```python
from build123d import *

# Parameters (mm, degrees)
SKETCH_1_W          = 80
SKETCH_1_H          = 50
EXTRUDE_1_DEPTH     = 2
SKETCH_5_W          = 2
SKETCH_5_H          = 50
EXTRUDE_2_DEPTH     = 2
SKETCH_2_W          = 30
SKETCH_2_H          = 4
SKETCH_2_W_2        = 35
SKETCH_2_H_2        = 16
CUT_EXTRUDE_1_DEPTH = 49.918299235
SKETCH_3_R          = 1.65
CUT_EXTRUDE_2_DEPTH = 49.918299235
SKETCH_6_W          = 1.5
SKETCH_6_H          = 4
CUT_EXTRUDE_4_DEPTH = 49.918299235
SKETCH_7_W          = 1.5
SKETCH_7_H          = 4
EXTRUDE_3_DEPTH     = 2
SKETCH_8_R          = 1.65
CUT_EXTRUDE_5_DEPTH = 49.918299235


with BuildPart() as part:
    # 草图1 → 凸台-拉伸1 (new body)
    with BuildSketch(Plane.XY):
        Rectangle(SKETCH_1_W, SKETCH_1_H)
    extrude(amount=EXTRUDE_1_DEPTH)

    # 草图5 → 凸台-拉伸2 (add)
    with BuildSketch(Plane.XY.offset(2)):
        with Locations((-41, 0)):
            Rectangle(SKETCH_5_W, SKETCH_5_H)
    extrude(amount=-EXTRUDE_2_DEPTH)

    # 草图2 → 切除-拉伸1 (cut, through all)
    with BuildSketch(Plane.XY.offset(2)):
        with Locations((0, -23)):
            Rectangle(SKETCH_2_W, SKETCH_2_H)
        with Locations((-0.5, -9)):
            Rectangle(SKETCH_2_W_2, SKETCH_2_H_2)
    extrude(amount=-CUT_EXTRUDE_1_DEPTH, mode=Mode.SUBTRACT)

    # 草图3 → 切除-拉伸2 (cut, through all)
    with BuildSketch(Plane.XY.offset(2)):
        with Locations((-39, -22)):
            Circle(SKETCH_3_R)
        with Locations((-19, -22)):
            Circle(SKETCH_3_R)
        with Locations(Location((17, -22, 0), (0, 0, 180))):
            Circle(SKETCH_3_R)
        with Locations(Location((37, -22, 0), (0, 0, 180))):
            Circle(SKETCH_3_R)
    extrude(amount=-CUT_EXTRUDE_2_DEPTH, mode=Mode.SUBTRACT)

    # 草图6 → 切除-拉伸4 (cut, through all)
    with BuildSketch(Plane.XY.offset(2)):
        with Locations((-15.75, -23)):
            Rectangle(SKETCH_6_W, SKETCH_6_H)
    extrude(amount=-CUT_EXTRUDE_4_DEPTH, mode=Mode.SUBTRACT)

    # 草图7 → 凸台-拉伸3 (add)
    with BuildSketch(Plane.XY.offset(2)):
        with Locations((14.25, -23)):
            Rectangle(SKETCH_7_W, SKETCH_7_H)
    extrude(amount=-EXTRUDE_3_DEPTH)

    # 草图8 → 切除-拉伸5 (cut, through all)
    with BuildSketch(Plane.XY.offset(2)):
        with Locations((-25, 11.5)):
            Circle(SKETCH_8_R)
        with Locations((-25, -8.5)):
            Circle(SKETCH_8_R)
        with Locations((25, -8.5)):
            Circle(SKETCH_8_R)
        with Locations((25, 11.5)):
            Circle(SKETCH_8_R)
    extrude(amount=-CUT_EXTRUDE_5_DEPTH, mode=Mode.SUBTRACT)


solid = part.part
```
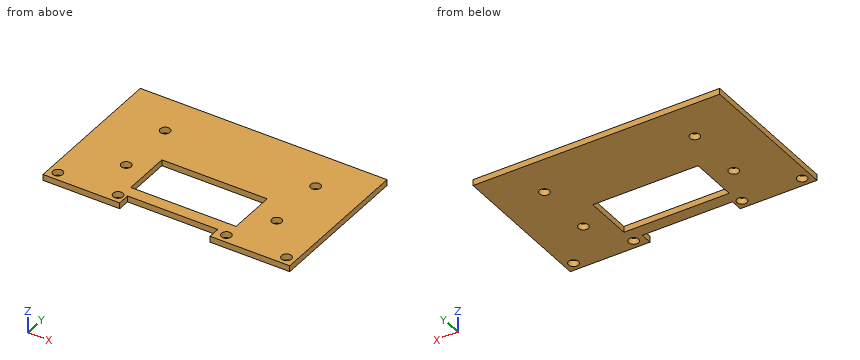
Work out the finished part from the listing and answer in its coordinate system (mm). Give positions to 0.01 mm unless a question says otherwise; leave off trailing zeros. Loops run counter-clockwise (first coordinate to the right, second up) from the corner with the lowest first, then second, coordinate; pieces in that order, holes last. Notation, with made-up numbers: (56, 83) -> (110, 83) arc R10 ccw to (110, 99) -> close; hole circle Ø11 at (17, -10). An arc over 180 degrees is marked (long way). Put each result on its own line as item: value. Start each with the question number.
Item 1: The part is cut by section C-C (z = 0.7). State how many separate pieces and enclosed holes the cut face has, then the cut area to 3 significant figures.
Item 2: Each of these flat-tipped pins is pushed along its axis until it touches: P1, Ø12, axis at x = 14, y = 12, coming from the -Z side; P2, Ø3, axis at x = -25, y = -8.5, coming from the +Z side; P3, Ø1, axis at x = 1, z = 1, coming from the -Y side. Where does it stop, or does it pass through?
Item 3: The part is cut by section D-D (y = -8.5). Give the vertices of the cut face in (x, z), then the cut area to 3 significant figures.
Item 4: Find the intervals of material crossed by L1, parallel to Y at x = -25, z = 1.2; L2, parallel to Y at x = 10, z = 1.1; L3, parallel to X at y = -3, z = 0.7, in increasing order. Write a range as [from, to].
Item 5: The part is cut by section A-A (y = -22). Give the vertices of the cut face in (x, z).
Item 6: The part is cut by section B-B (x = 25). Give the vertices of the cut face in (y, z).
Answers below:
1. separate pieces: 1
1. enclosed holes: 9
1. area: 3,350 mm2
2. P1: z = 0
2. P2: through
2. P3: y = -21
3. outline: (-42, 0) -> (-26.65, 0) -> (-26.65, 2) -> (-42, 2) -> close; (-23.35, 0) -> (-18, 0) -> (-18, 2) -> (-23.35, 2) -> close; (17, 0) -> (23.35, 0) -> (23.35, 2) -> (17, 2) -> close; (26.65, 0) -> (40, 0) -> (40, 2) -> (26.65, 2) -> close
3. area: 80.8 mm2
4. L1: [-25, -10.15], [-6.85, 9.85], [13.15, 25]
4. L2: [-21, -17], [-1, 25]
4. L3: [-42, -18], [17, 40]
5. outline: (-42, 0) -> (-40.65, 0) -> (-40.65, 2) -> (-42, 2) -> close; (-37.35, 0) -> (-20.65, 0) -> (-20.65, 2) -> (-37.35, 2) -> close; (-17.35, 0) -> (-16.5, 0) -> (-16.5, 2) -> (-17.35, 2) -> close; (13.5, 0) -> (15.35, 0) -> (15.35, 2) -> (13.5, 2) -> close; (18.65, 0) -> (35.35, 0) -> (35.35, 2) -> (18.65, 2) -> close; (38.65, 0) -> (40, 0) -> (40, 2) -> (38.65, 2) -> close
6. outline: (-25, 0) -> (-10.15, 0) -> (-10.15, 2) -> (-25, 2) -> close; (-6.85, 0) -> (9.85, 0) -> (9.85, 2) -> (-6.85, 2) -> close; (13.15, 0) -> (25, 0) -> (25, 2) -> (13.15, 2) -> close
